Can you work these out from the model? Positions are in its coordinate system, mm. Face numbers are marked on the shaded views. A direction names the side the tool comes from. Round coordinates to 2 decimals unless told otherwise and drop trailing zeros. Loops run counter-clockwise (first coordinate to the right, second up) from the corner with the lowest first, then second, coordinate; pieces in that order, holes last.
from build123d import *

# Parameters (mm, degrees)
F0_W      = 43.18
F0_H      = 38.1
F0_W_2    = 38.1
F0_H_2    = 33.02
F1_DEPTH  = 44.45
F2_W      = 38.1
F2_H      = 33.02
F2_R      = 2.159
F3_DEPTH  = 25.4
F4_R      = 2.159
F5_DEPTH  = 5.08
F6_R      = 3.175
F7_DEPTH  = 16.256
F8_R      = 5.08
F9_DEPTH  = 11.938
F10_R     = 5.334
F11_DEPTH = 11.938


with BuildPart() as f1:
    # F0 (on Top) → F1 (new body, symmetric)
    with BuildSketch(Plane.XY):
        Rectangle(F0_W, F0_H)
        Rectangle(F0_W_2, F0_H_2, mode=Mode.SUBTRACT)
    extrude(amount=F1_DEPTH, both=True)

    # F2 (on face) → F3 (join)
    with BuildSketch(Plane.XY.offset(44.45)):
        Rectangle(F2_W, F2_H)
        with Locations((-6.35, 0)):
            Circle(F2_R, mode=Mode.SUBTRACT)
        with Locations((6.35, 0)):
            Circle(F2_R, mode=Mode.SUBTRACT)
    extrude(amount=-F3_DEPTH)

    # F4 (on face) → F5 (cut)
    with BuildSketch(Plane(origin=(0, 0, 19.05), x_dir=(1, 0, 0), z_dir=(0, 0, -1))):
        Polygon((9.017, 4.6193795038), (3.683, 4.6193795038), (1.016, 0), (3.683, -4.6193795038), (9.017, -4.6193795038), (11.684, 0), align=None)
        with Locations((6.35, 0)):
            Circle(F4_R, mode=Mode.SUBTRACT)
        Polygon((-3.683, 4.6193795038), (-9.017, 4.6193795038), (-11.684, 0), (-9.017, -4.6193795038), (-3.683, -4.6193795038), (-1.016, 0), align=None)
        with Locations((-6.35, 0)):
            Circle(F4_R, mode=Mode.SUBTRACT)
    extrude(amount=-F5_DEPTH, mode=Mode.SUBTRACT)

    # F6 (on face) → F7 (cut)
    with BuildSketch(Plane.XZ.offset(19.05)):
        with Locations((0, 11.43)):
            Circle(F6_R)
        with Locations((0, 1.778)):
            Circle(F6_R)
        with Locations((0, -7.874)):
            Circle(F6_R)
        with Locations((0, -17.526)):
            Circle(F6_R)
        with Locations((0, -27.178)):
            Circle(F6_R)
        with Locations((0, -36.83)):
            Circle(F6_R)
    extrude(amount=-F7_DEPTH, mode=Mode.SUBTRACT)

    # F8 (on face) → F9 (cut)
    with BuildSketch(Plane(origin=(-21.59, 0, 0), x_dir=(0, -1, 0), z_dir=(-1, 0, 0))):
        with Locations((0, 34.29)):
            Circle(F8_R)
    extrude(amount=-F9_DEPTH, mode=Mode.SUBTRACT)

    # F10 (on face) → F11 (cut)
    with BuildSketch(Plane.YZ.offset(21.59)):
        with Locations((0, 34.29)):
            Circle(F10_R)
    extrude(amount=-F11_DEPTH, mode=Mode.SUBTRACT)


solid = f1.part
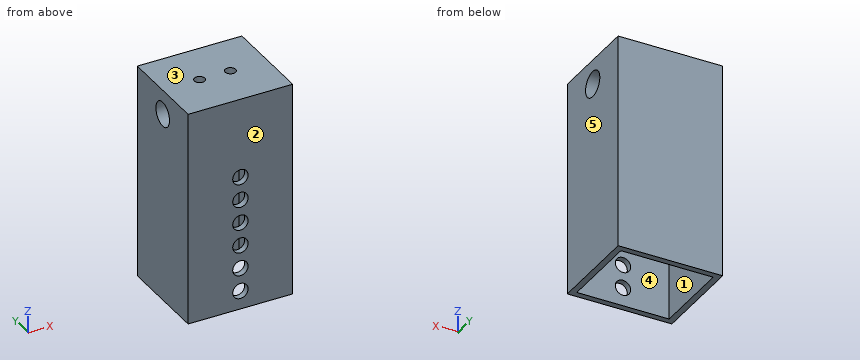
(1) For the marked faces 4 and 5, which set-ups out of +Z, -Z, +X, -X, +Y, -Y let a thin tool reach every point of the face, with its end or its side?
Worked answers:
face 4: -Z
face 5: +Z, -Z, +X, +Y, -Y
(2) If we section it at A-A, the plane x = 0: State how many separate pieces and enclosed holes the cut face has, then the cut area to 3 significant figures.
Worked answers:
separate pieces: 7
enclosed holes: 0
area: 1,190 mm2
(3) If we section it at C-C, the plane z = 11.43: List the corners of the cut face in (x, y) for me (3 decimals).
Worked answers:
outline: (-21.59, -19.05) - (-3.175, -19.05) - (-3.175, -16.51) - (-19.05, -16.51) - (-19.05, 16.51) - (19.05, 16.51) - (19.05, -16.51) - (3.175, -16.51) - (3.175, -19.05) - (21.59, -19.05) - (21.59, 19.05) - (-21.59, 19.05) - close
(4) If I drill on line 1 (X direction, y = 0, z = 33); line 2 (X direction, y = 15.5, z = -33); line 3 (Z direction, x = -15, y = 0), over which ranges is the centre line in solid material (lowest first)?
Worked answers:
line 1: x = -9.65 to -8.51, -4.19 to 4.19, 8.51 to 9.65
line 2: x = -21.59 to -19.05, 19.05 to 21.59
line 3: z = 19.05 to 29.21, 39.37 to 44.45
(5) Will these pins go through, and if not, where does the flat tip stop? P1, Ø3, axis at y = -1, z = 32.5, coming from the +X side; P2, Ø10, axis at x = 8.5, y = -2, coming from the -Z side; P3, Ø12, axis at x = 17, y = 4, coming from the -Z side; P4, Ø7, axis at x = 6.35, y = 0, coming from the -Z side.
Worked answers:
P1: stops at x = 9.65
P2: stops at z = 19.05
P3: stops at z = -44.45
P4: stops at z = 24.13
(6) If we mould it in two halves opening along Y, with no side actions, what happens to the marked faces 1, 2 and 3? For each: released by +Y, released by -Y, zero draft, split by the parting line, or undercut.
Worked answers:
face 1: undercut
face 2: released by -Y
face 3: zero draft
(7) If we section it at B-B, the plane y = 7.5: List the corners of the cut face in (x, z) for me, then the cut area to 3 significant figures.
Worked answers:
outline: (-21.59, -44.45) - (-19.05, -44.45) - (-19.05, 19.05) - (19.05, 19.05) - (19.05, -44.45) - (21.59, -44.45) - (21.59, 44.45) - (-21.59, 44.45) - close
area: 1,420 mm2
(8) If we section it at D-D, the plane x = 6.35: List the corners of the cut face in (y, z) for me.
Worked answers:
outline: (-19.05, -44.45) - (-16.51, -44.45) - (-16.51, 19.05) - (-4.62, 19.05) - (-4.62, 24.13) - (-2.16, 24.13) - (-2.16, 44.45) - (-19.05, 44.45) - close; (2.16, 24.13) - (4.62, 24.13) - (4.62, 19.05) - (16.51, 19.05) - (16.51, -44.45) - (19.05, -44.45) - (19.05, 44.45) - (2.16, 44.45) - close
